Geometry check sheet. Reference: drawing and pictorial views, mm from the part's lowest x, y, z. Coordinates: 2 decimals unless noted, no trailing zeros. Order: outer loops, then holes, each group sorted by start corner. A loop starts at its lowest first (then second) coordinate and runs counter-clockwise, first axis right, second up. Notation, with made-up numbers: M 47,71 L 104,71 A13 ccw 104,75 Z; hole C 68.25,39 d7. An arc over 180 degrees is marked long. Return JSON: item names as keys, results as strings.
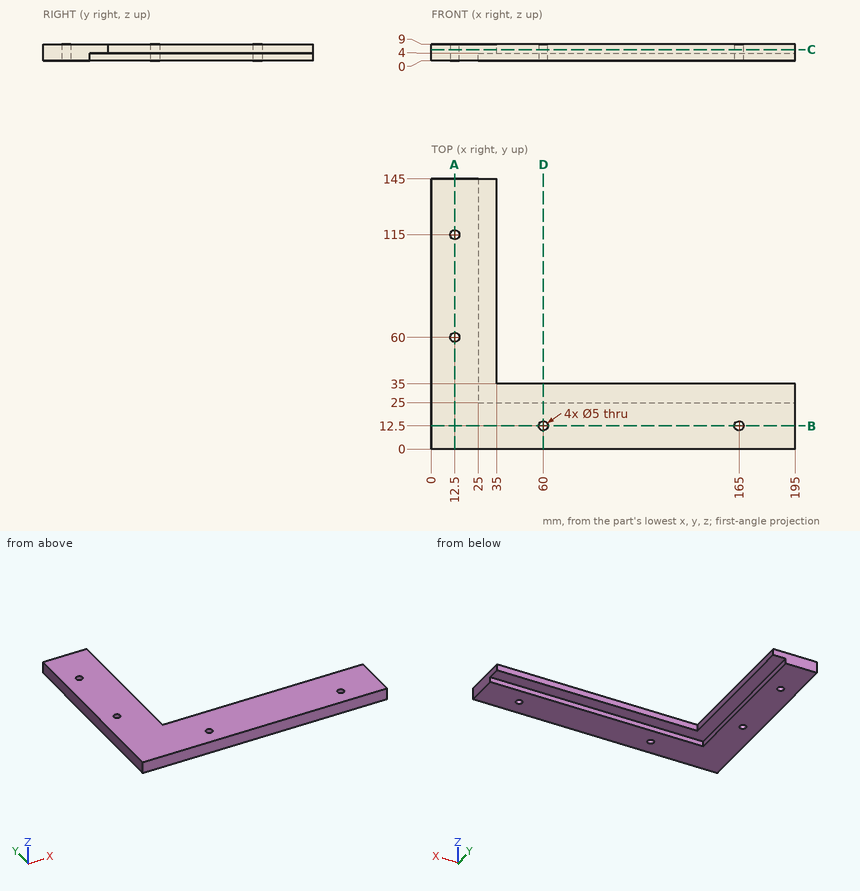
Q1. Cross-section at B-B, the plane y = 12.5. Record the boundary of the cut face in (x, z).
Values:
{"outline": "M 0,0 L 57.5,0 L 57.5,9 L 0,9 Z; M 62.5,0 L 162.5,0 L 162.5,9 L 62.5,9 Z; M 167.5,0 L 195,0 L 195,9 L 167.5,9 Z"}
Q2. Go/stop test with flat-tipped pins: pin 1 (4 mm diameter, centred on x = 126, z = 3.5, fed in from +Y); pin 2 (3 mm diameter, centred on y = 57.5, z = 1.5, fed in from +X); pin 3 (2.5 mm diameter, centred on y = 95.5, z = 7, fed in from +X); pin 4 (4 mm diameter, centred on x = 165, y = 12.5, fed in from -Z). Record where each tip stops, or that it passes through.
Values:
{"pin 1": "y = 35", "pin 2": "x = 25", "pin 3": "x = 35", "pin 4": "through"}
Q3. Material ranges on line 1 along X through (y, z) = (12.5, 4.75); line 2 along Y through (x, z) = (12.5, 4); line 3 along X through (y, z) = (115, 7.25), recorded low to high.
Values:
{"line 1": "0 to 57.5, 62.5 to 162.5, 167.5 to 195", "line 2": "0 to 57.5, 62.5 to 112.5, 117.5 to 145", "line 3": "0 to 10, 15 to 35"}
Q4. Cross-section at A-A, the plane x = 12.5. Record the boundary of the cut face in (y, z).
Values:
{"outline": "M 0,0 L 57.5,0 L 57.5,9 L 0,9 Z; M 62.5,0 L 112.5,0 L 112.5,9 L 62.5,9 Z; M 117.5,0 L 145,0 L 145,9 L 117.5,9 Z"}
Q5. Cross-section at D-D, the plane x = 60. Record the boundary of the cut face in (y, z), and give its area (3 significant figures).
Values:
{"outline": "M 0,0 L 10,0 L 10,9 L 0,9 Z; M 15,0 L 25,0 L 25,4 L 35,4 L 35,9 L 15,9 Z", "area": "230 mm^2"}
Q6. Cross-section at C-C, the plane z = 6. Record the boundary of the cut face in (x, y), and give its area (3 significant figures).
Values:
{"outline": "M 0,0 L 195,0 L 195,35 L 35,35 L 35,145 L 0,145 Z; hole C 12.5,60 d5; hole C 12.5,115 d5; hole C 60,12.5 d5; hole C 165,12.5 d5", "area": "10,600 mm^2"}
